Check sheet for the modelled part. Datum: model origin and axes. Units: mm. A direction names the side the tool comes from. Give positions to 0.01 mm unless a question says otherwise; leave off trailing zeros. Order: outer loops, then holes, each group sorted by start corner. A loop starts at its lowest first (then second) coordinate and runs counter-clockwise, first axis right, second up. Notation, with made-up numbers: M -7.5,68 L -3.5,68 A5 cw -3.5,77 Z; hole C 80.5,61 d7. An arc over 180 degrees is marked long. Answer in a Markdown table with one row per item. Add a question column.
from build123d import *

# Parameters (mm, degrees)
SKETCH1_W                   = 50.8
SKETCH1_H                   = 25.4
SKETCH1_W_2                 = 44.45
SKETCH1_H_2                 = 19.05
BOSS_EXTRUDE1_DEPTH         = 355.6
CUT_EXTRUDE1_DEPTH          = 361.10715072
CUT_EXTRUDE1_DEPTH_BACK     = 361.10715072
SKETCH2_R                   = 3.175
F_1_4_0_25_DIAMETER_HOLE1_D = 6.35


with BuildPart() as part:
    # Sketch1 → Boss-Extrude1 (new body)
    with BuildSketch(Plane.XY):
        with Locations((25.4, 12.7)):
            Rectangle(SKETCH1_W, SKETCH1_H)
        with Locations((25.4, 12.7)):
            Rectangle(SKETCH1_W_2, SKETCH1_H_2, mode=Mode.SUBTRACT)
    extrude(amount=BOSS_EXTRUDE1_DEPTH)

    # Sketch2 → Cut-Extrude1 (cut, two sides: drawn at the far end of the back side and taken through both)
    with BuildSketch(Plane.ZY.offset(-CUT_EXTRUDE1_DEPTH_BACK)):
        with Locations((133.35, 12.7)):
            Circle(SKETCH2_R)
        with Locations((146.05, 12.7)):
            Circle(SKETCH2_R)
        with Locations((95.25, 12.7)):
            Circle(SKETCH2_R)
        with Locations((57.15, 12.7)):
            Circle(SKETCH2_R)
        with Locations((209.55, 12.7)):
            Circle(SKETCH2_R)
        with Locations((222.25, 12.7)):
            Circle(SKETCH2_R)
        with Locations((260.35, 12.7)):
            Circle(SKETCH2_R)
        with Locations((298.45, 12.7)):
            Circle(SKETCH2_R)
    extrude(amount=CUT_EXTRUDE1_DEPTH + CUT_EXTRUDE1_DEPTH_BACK, mode=Mode.SUBTRACT)

    # 1/4 (0.25) Diameter Hole1 (through all)
    with Locations(Plane(origin=(0, 25.4, 0), x_dir=(1, 0, 0), z_dir=(0, 1, 0))):
        with Locations((12.7, -12.7), (25.4, -12.7), (38.1, -12.7), (12.7, -342.9), (25.4, -342.9), (38.1, -342.9)):
            Hole(F_1_4_0_25_DIAMETER_HOLE1_D / 2)


solid = part.part
Q1. Cross-section at B-B (z = 95.25). Record the boundary of the cut face in (x, y) (3 decimals), and give its area (3 significant figures).
Q2. Cross-section at A-A (x = 12.7). Record the boundary of the cut face in (y, z) (3 decimals), and give its area (3 significant figures).
Q3. Cross-section at C-C (x = 31.5). Record the boundary of the cut face in (y, z) (3 decimals).
Q4. Thickness scan on probe 1 along Y at (x, z) = (26.5, 227.5) (3 decimals); probe 2 along X at (y, z) = (8.25, 298.5) (3 decimals); probe 3 along Y at (x, z) = (2, 298). Record the ranges inside material, lowest first.
Q5. Go/stop test with a flat-tipped pin: pin 1 (8.5 mm diameter, centred on y = 12.7, z = 209.55, fed in from +X). Record where the tip stops, or that it passes through.
Q6. Tool access check on faces 1 (the flat face through (25, 3.175, 175)), 2 (the cylindrical face through (38.51, 23.79, 339.75)). Record the directions out of +Z, -Z, +X, -X, +Y, -Y that give a thin tool (end or side, any length) a straight path to the whole face; none if there is none.
Q7. Draft check along X on faces 3 (the flat face through (50.8, 13, 175)), 4 (the cylindrical face through (49.23, 12.84, 219.08)), 5 (the cylindrical face through (41.27, 1.57, 12.56)). Enter one of: pulls with the +X half, pulls with the -X half, needs draft (parallel to the pull), parting line crosses it, or undercut.
Values follow:
| question | item | result |
|---|---|---|
| 1 | outline | M 0,0 L 50.8,0 L 50.8,9.525 L 47.625,9.525 L 47.625,3.175 L 3.175,3.175 L 3.175,9.525 L 0,9.525 Z; M 0,15.875 L 3.175,15.875 L 3.175,22.225 L 47.625,22.225 L 47.625,15.875 L 50.8,15.875 L 50.8,25.4 L 0,25.4 Z |
| 1 | area | 403 mm² |
| 2 | outline | M 0,0 L 3.175,0 L 3.175,9.525 L 0,9.525 Z; M 0,15.875 L 3.175,15.875 L 3.175,339.725 L 0,339.725 Z; M 0,346.075 L 3.175,346.075 L 3.175,355.6 L 0,355.6 Z; M 22.225,0 L 25.4,0 L 25.4,9.525 L 22.225,9.525 Z; M 22.225,15.875 L 25.4,15.875 L 25.4,339.725 L 22.225,339.725 Z; M 22.225,346.075 L 25.4,346.075 L 25.4,355.6 L 22.225,355.6 Z |
| 2 | area | 2,180 mm² |
| 3 | outline | M 0,0 L 3.175,0 L 3.175,355.6 L 0,355.6 Z; M 22.225,0 L 25.4,0 L 25.4,355.6 L 22.225,355.6 Z |
| 4 | probe 1 | 0 to 3.175, 22.225 to 25.4 |
| 4 | probe 2 | 0 to 3.175, 47.625 to 50.8 |
| 4 | probe 3 | 0 to 9.56, 15.84 to 25.4 |
| 5 | pin 1 | x = 50.8 |
| 6 | face 1 | +Z, -Z |
| 6 | face 2 | +Y, -Y |
| 7 | face 3 | pulls with the +X half |
| 7 | face 4 | needs draft |
| 7 | face 5 | undercut |
